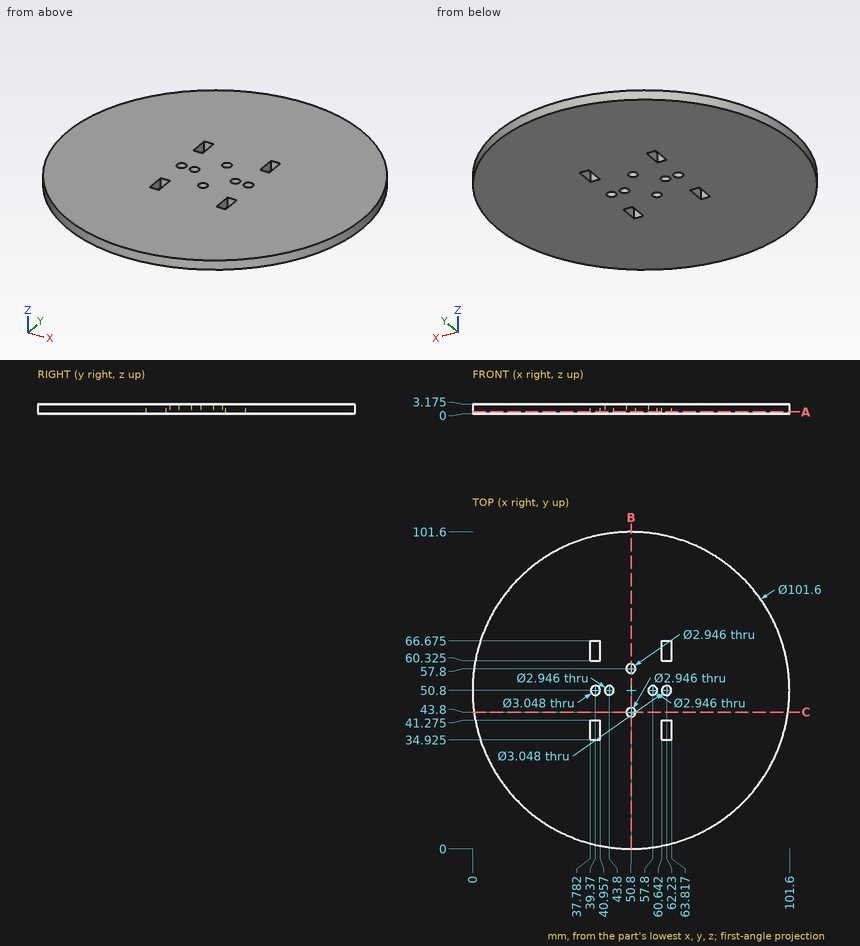
Geometry check sheet. Reference: drawing and pictorial views, mm from the part's lowest x, y, z. Coordinates: 2 decimals unless noted, no trailing zeros. Order: outer loops, then holes, each group sorted by start corner. A loop starts at its lowest first (then second) coordinate and runs counter-clockwise, first axis right, second up. Notation, with made-up numbers: (53.25, 34.25) -> (107.25, 34.25) arc R13 cw to (107.25, 59.25) -> close; hole circle Ø6 at (60, -20). An arc over 180 degrees is marked (long way). Put each result on its own line as item: value. Start each with the question number.
1) Go/stop test with flat-tipped pins: pin 1 (1 mm diameter, centred on x = 39.5, z = 1, fed in from -Y); pin 2 (1.6 mm diameter, centred on y = 39.5, z = 1, fed in from -X); pin 3 (1 mm diameter, centred on x = 44, z = 1, fed in from +Y). Record where each tip stops, or that it passes through.
2) Cross-section at C-C (y = 43.8). Enter the section's corners in (x, z) (1 decimal).
3) Cross-section at B-B (x = 50.8). Enter the section's corners in (y, z) (1 decimal), plus the area to 3 significant figures.
4) Cross-section at A-A (z = 0.65). State how many separate pieces and enclosed holes the cut face has.
5) Material ranges on L1, parallel to Y at x = 50.8, z = 2.15; L2, parallel to Y at x = 39.37, z = 1.55 (1 decimal); L3, parallel to Y at x = 43.8, z = 1.95 (1 decimal), recorded low to high.
Geometry check:
1. pin 1: stops at y = 1.16
1. pin 2: stops at x = 1.1
1. pin 3: stops at y = 101.21
2. outline: (0.5, 0) -> (49.3, 0) -> (49.3, 3.2) -> (0.5, 3.2) -> close; (52.3, 0) -> (101.1, 0) -> (101.1, 3.2) -> (52.3, 3.2) -> close
3. outline: (0, 0) -> (42.3, 0) -> (42.3, 3.2) -> (0, 3.2) -> close; (45.3, 0) -> (56.3, 0) -> (56.3, 3.2) -> (45.3, 3.2) -> close; (59.3, 0) -> (101.6, 0) -> (101.6, 3.2) -> (59.3, 3.2) -> close
3. area: 304 mm^2
4. separate pieces: 1
4. enclosed holes: 10
5. L1: y = 0 to 42.33, 45.27 to 56.33, 59.27 to 101.6
5. L2: y = 1.3 to 34.9, 41.3 to 49.3, 52.3 to 60.3, 66.7 to 100.3
5. L3: y = 0.5 to 49.3, 52.3 to 101.1
